Input: dimensioned drawing with shaded views. Units: mm. Origin: part minimum x, y, z. Round coordinates to 2 decimals unless told otherwise and drop trailing zeros. Loops run counter-clockwise (first coordinate to the right, second up) from the corner with the lowest first, then second, coordinate; pieces in that order, holes last. Notation, with made-up numbers: M 14,39.5 L 42,39.5 A23 ccw 42,60.5 Z; hole C -4.5,13.25 d11. An arc over 180 degrees is marked long. Answer as a JSON object with one key per item and string values.
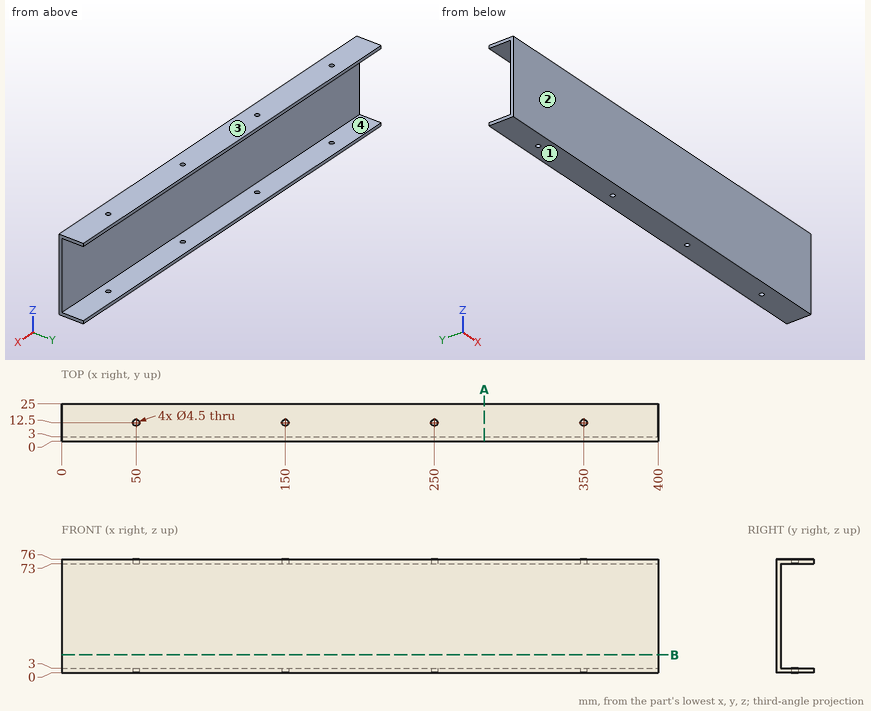
Item 1: Pull-direction query (Z, two-part tool) for the marked faces 1, 2, 3 and 4; classes: pulls with the +Z half, pulls with the -Z half, needs draft (parallel to the pull), parting line crosses it, or undercut.
Answer sheet:
{"face 1": "pulls with the -Z half", "face 2": "needs draft", "face 3": "pulls with the +Z half", "face 4": "undercut"}
Item 2: Line query: probe 1 along Z at (x, y) = (82.5, 3.75); probe 2 along Y at (x, z) = (350, 74); probe 3 along Y at (x, z) = (383, 64). Output: solid intervals per line, ascending. Write a range as from..to.
Answer sheet:
{"probe 1": "z = 0..3, 73..76", "probe 2": "y = 0..10.25, 14.75..25", "probe 3": "y = 0..3"}
Item 3: Section A-A on x = 283.5. Return the cut outline in (y, z), then the cut area to 3 significant figures.
Answer sheet:
{"outline": "M 0,0 L 25,0 L 25,3 L 3,3 L 3,73 L 25,73 L 25,76 L 0,76 Z", "area": "360 mm²"}
Item 4: Section B-B on z = 12. Return the cut outline in (x, y).
Answer sheet:
{"outline": "M 0,0 L 400,0 L 400,3 L 0,3 Z"}
Item 5: Contact query for flat-ended pins moving along their axis: pin 1 Ø6 at (x, y) = (350, 12.5) entering from -Z; pin 2 Ø3.5 at (x, y) = (350, 12.5) entering from +Z; pin 3 Ø21 at (x, z) = (153, 23) entering from +Y. Output: stop coordinate, or through.
Answer sheet:
{"pin 1": "stops at z = 0", "pin 2": "passes through", "pin 3": "stops at y = 3"}
